Here's the drawing with two shaded views (mm, measured from the low corner). I have some questions. A direction names the side the tool comes from. Coordinates: 2 decimals unless noted, no trailing zeros. Write each loop counter-clockwise with the first axis right and the second up, starting at its lowest first coordinate (ties: lowest second). Pieces come first, ordered by that corner, then holes. Notation, with made-up numbers: M -16.5,-34.5 L -2.5,-34.5 A27 cw -2.5,-8.5 Z; hole C 88.25,80.5 d9. An arc over 180 degrees is marked long. Answer as CSV lines item,"result". Start each with the question number.
Item 1: Suppose I cut it at B-B, the plane x = 18. Write out the boundary of the cut face in (y, z) (1 decimal), and give its area (3 significant figures).
Item 2: I'm going to push flat-ended pins straight in: P1, Ø1.5, axis at x = 14, z = 39.5, coming from the +Y side; P2, Ø2, axis at y = 49.5, z = 19.5, coming from the +X side; P3, Ø4, axis at x = 47.5, z = 57.5, coming from the -Y side (3 decimals). Where does each tip first touch, or does it pass through?
Item 3: Suppose I cut it at C-C, the plane z = 6. Write out the boundary of the cut face in (x, y).
Item 4: On a 3-axis mill with a long thin cutter (end or side, diameter ignored), from which of +Z, -Z, +X, -X, +Y, -Y can I reach the whole of each face in a straight line? I mean the marked faces 1, 2 and 3. Say none if no direction works.
Item 5: If I drill on line 1 along X through (y, z) = (52.5, 33.5); line 2 along Z through (x, y) = (55.5, 39.5); line 3 along Y through (x, z) = (52, 56.5) (1 decimal), over which ranges is the centre line in solid material (lowest first)? Write a range as [from, to].
Item 6: Suppose I cut it at A-A, the plane y = 32. Write out the boundary of the cut face in (x, z), and give its area (3 significant figures).
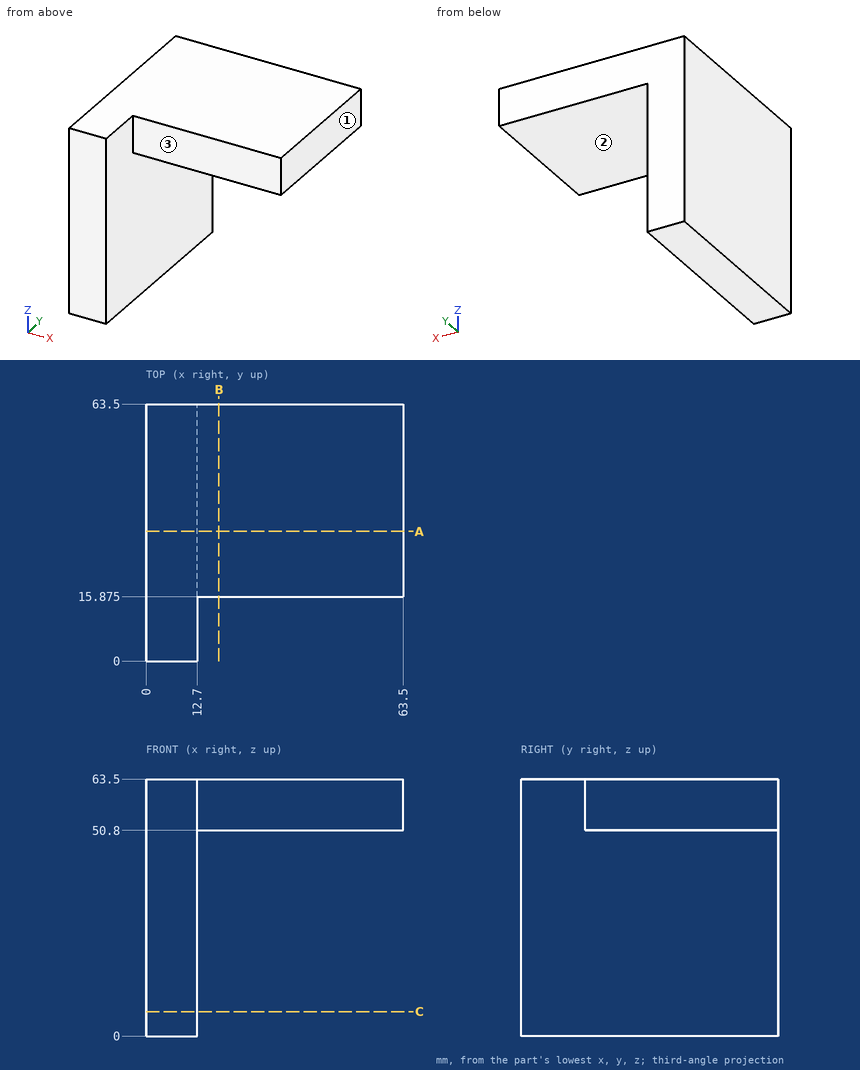
Ans:
1,outline,"M 15.9,50.8 L 63.5,50.8 L 63.5,63.5 L 15.9,63.5 Z"
1,area,"605 mm^2"
2,P1,"passes through"
2,P2,"stops at x = 12.7"
2,P3,"stops at y = 15.875"
3,outline,"M 0,0 L 12.7,0 L 12.7,63.5 L 0,63.5 Z"
4,face 1,"+Z, -Z, +X, +Y, -Y"
4,face 2,"-Z, +X, +Y, -Y"
4,face 3,"+Z, -Z, +X, -Y"
5,line 1,"x = [0, 12.7]"
5,line 2,"z = [50.8, 63.5]"
5,line 3,"y = [15.9, 63.5]"
6,outline,"M 0,0 L 12.7,0 L 12.7,50.8 L 63.5,50.8 L 63.5,63.5 L 0,63.5 Z"
6,area,"1,450 mm^2"
